```python
from build123d import *

# Parameters (mm, degrees)
SKETCH1_R                = 7.9375
SKETCH1_R_2              = 6.35
BOSS_EXTRUDE1_DEPTH      = 76.2
BOSS_EXTRUDE2_START      = -3.175
SKETCH2_R                = 15.875
SKETCH2_R_2              = 6.35
BOSS_EXTRUDE2_DEPTH      = 3.175
M3_CLEARANCE_HOLE1_D     = 3.4
M3_CLEARANCE_HOLE1_DEPTH = 4
M3_CLEARANCE_HOLE1_TIP   = 1.021463052


with BuildPart() as part:
    # Sketch1 → Boss-Extrude1 (new body)
    with BuildSketch(Plane.XY):
        with Locations(Location((0, 0, 0), (0, 0, 180))):
            Circle(SKETCH1_R)
        with Locations(Location((0, 0, 0), (0, 0, 180))):
            Circle(SKETCH1_R_2, mode=Mode.SUBTRACT)
    extrude(amount=BOSS_EXTRUDE1_DEPTH)

    # Sketch2 → Boss-Extrude2 (add)
    with BuildSketch(Plane.XY.offset(76.2).offset(BOSS_EXTRUDE2_START)):
        Circle(SKETCH2_R)
        with Locations(Location((0, 0, 0), (0, 0, 180))):
            Circle(SKETCH2_R_2, mode=Mode.SUBTRACT)
    extrude(amount=BOSS_EXTRUDE2_DEPTH)

    # M3 Clearance Hole1
    with Locations(Plane.XY.offset(76.2)):
        with Locations((0, 12.7), (0, -12.7), (12.7, 0), (-12.7, 0)):
            Hole(M3_CLEARANCE_HOLE1_D / 2, depth=M3_CLEARANCE_HOLE1_DEPTH)
            with Locations((0, 0, -(M3_CLEARANCE_HOLE1_DEPTH + M3_CLEARANCE_HOLE1_TIP / 2))):  # 118° drill point
                Cone(0, M3_CLEARANCE_HOLE1_D / 2, M3_CLEARANCE_HOLE1_TIP, mode=Mode.SUBTRACT)


solid = part.part
```
Check sheet for the modelled part. Datum: model origin and axes. Units: mm. A direction names the side the tool comes from. Round coordinates to 2 decimals unless told otherwise and drop trailing zeros. Order: outer loops, then holes, each group sorted by start corner. A loop starts at its lowest first (then second) coordinate and runs counter-clockwise, first axis right, second up.
1) Go/stop test with flat-tipped pins: pin 1 Ø4.5 at (x, y) = (0, -12.7) entering from -Z (3 decimals); pin 2 Ø6 at (y, z) = (6, 60) entering from +X; pin 3 Ø8 at (y, z) = (-6.5, 21.5) entering from -X. Record where each tip stops, or that it passes through.
2) Section check B-B (y = 0). Give the number of separate pieces and of enclosed holes in the cut face, and give its area (3 significant figures).
3) Section check A-A (x = -13). Record the boundary of the cut face in (y, z) (3 decimals).
4) Scan lines: line 1 (Y direction, x = 0, z = 21); line 2 (Y direction, x = 0, z = 75.2) (3 decimals); line 3 (Z direction, x = -13, y = 7.5) (3 decimals). Record each from-to range of solid material in increasing order.
5) Section check C-C (y = 12.7). Record the boundary of the cut face in (x, z) (3 decimals).
6) Tool access check on faces 5 (the cylindrical face through (0, -11, 75)), 6 (the flat face through (-3.8, 7.3, 73.025)). Record the directions out of +Z, -Z, +X, -X, +Y, -Y that give a thin tool (end or side, any length) a straight path to the whole face; none if there is none.
7) Mould release check, pull along X, two halves, no side actions. Record for faces 1 (the flat face through (0, -7, 0)), 2 (the cylindrical face through (-2.93, 5.634, 37.567)), 3 (the cylindrical face through (1.72, 7.75, 36)), 4 (the cylindrical face through (14.05, -1.03, 74.59)): +X half, -X half, draft (parallel to the pull), parting line (faces both ways), or undercut.
Result:
1. pin 1: stops at z = 73.025
1. pin 2: stops at x = 7.35
1. pin 3: stops at x = -7.53
2. separate pieces: 4
2. enclosed holes: 0
2. area: 271 mm2
3. outline: (-9.111, 73.025) - (-1.673, 73.025) - (-1.673, 76.2) - (-9.111, 76.2) - close; (1.673, 73.025) - (9.111, 73.025) - (9.111, 76.2) - (1.673, 76.2) - close
4. line 1: y = -7.94 to -6.35, 6.35 to 7.94
4. line 2: y = -15.875 to -14.4, -11 to -6.35, 6.35 to 11, 14.4 to 15.875
4. line 3: z = 73.025 to 76.2
5. outline: (-9.525, 73.025) - (-1.7, 73.025) - (-1.7, 76.2) - (-9.525, 76.2) - close; (1.7, 73.025) - (9.525, 73.025) - (9.525, 76.2) - (1.7, 76.2) - close
6. face 5: +Z, -Z
6. face 6: -Z
7. face 1: draft
7. face 2: undercut
7. face 3: parting line
7. face 4: undercut
